Check sheet for the modelled part. Datum: model origin and axes. Units: mm. Face numbers are marked on the shaded views. A direction names the side the tool comes from. Round coordinates to 2 decimals unless told otherwise and drop trailing zeros. Loops run counter-clockwise (first coordinate to the right, second up) from the corner with the lowest first, then second, coordinate; pieces in that order, holes last. Notation, with made-up numbers: (83, 42) - (137, 42) arc R17 ccw to (137, 48) - close; hole circle Ø8 at (-35.5, 25). An arc over 180 degrees is marked (long way). Return JSON: item names as keys, results as strings.
Autodesk Inventor part; units mm, degrees
ref_plane "YZ Plane" through (0, 0, 0) normal (1, 0, 0) x (0, 1, 0)
ref_plane "XZ Plane" through (0, 0, 0) normal (0, 1, 0) x (-1, 0, 0)
ref_plane "XY Plane" through (0, 0, 0) normal (0, 0, 1) x (1, 0, 0)
sketch "Sketch1" plane through (0, 0, 0) normal (0, 0, 1) x (1, 0, 0)
  circle A0 centre (0, 0) radius 3
  dimension "d0" = 6
extrude "Extrusion1" add sketch "Sketch1" along normal blind 0.5
sketch "Sketch2" plane through (0, 0, 0.5) normal (0, 0, 1) x (1, 0, 0)
  circle A0 centre (0, 0) radius 3
  circle A1 centre (0, 0) radius 2
  dimension "d3" = 4
extrude "Extrusion2" add sketch "Sketch2" along normal blind 3 contours A1
hole "Hole1" at (0, 0, 3.5) direction (0, 0, -1) diameter 2 depth 3.5
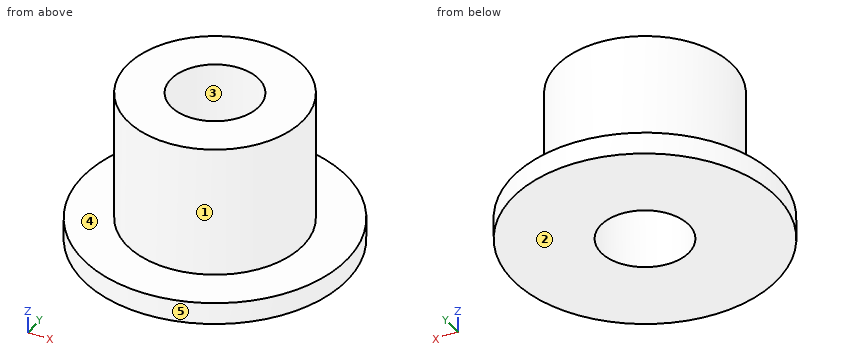
Q1. Tool access check on the marked faces 4 and 5. Record the directions out of +Z, -Z, +X, -X, +Y, -Y that give a thin tool (end or side, any length) a straight path to the whole face; none if there is none.
Answer key:
{"face 4": "+Z", "face 5": "+Z, -Z"}
Q2. Sectioned sample at B-B (y = 0.3). Enter the section's corners in (x, z), plus the area to 3 significant figures.
Answer key:
{"outline": "(-2.98, 0) - (-0.95, 0) - (-0.95, 3.5) - (-1.98, 3.5) - (-1.98, 0.5) - (-2.98, 0.5) - close; (0.95, 0) - (2.98, 0) - (2.98, 0.5) - (1.98, 0.5) - (1.98, 3.5) - (0.95, 3.5) - close", "area": "8.17 mm²"}
Q3. Sectioned sample at D-D (x = 1.9). Enter the section's corners in (y, z), plus the area to 3 significant figures.
Answer key:
{"outline": "(-2.32, 0) - (2.32, 0) - (2.32, 0.5) - (0.62, 0.5) - (0.62, 3.5) - (-0.62, 3.5) - (-0.62, 0.5) - (-2.32, 0.5) - close", "area": "6.07 mm²"}
Q4. Draft check along X on the marked faces 1, 2 and 3. Enter one of: released by +X, released by -X, zero draft, split by the parting line, or undercut.
Answer key:
{"face 1": "split by the parting line", "face 2": "zero draft", "face 3": "undercut"}
Q5. Scan lines: probe 1 along Y at (x, z) = (0, 2.7); probe 2 along Z at (x, y) = (-2, -2.2); probe 3 along X at (y, z) = (0.4, 2.5). Record each from-to range of solid material in increasing order. Write a range as [from, to].
Answer key:
{"probe 1": "y = [-2, -1], [1, 2]", "probe 2": "z = [0, 0.5]", "probe 3": "x = [-1.96, -0.92], [0.92, 1.96]"}
Q6. Sectioned sample at C-C (y = 1.35). Enter the section's corners in (x, z), plus the area to 3 significant figures.
Answer key:
{"outline": "(-2.68, 0) - (2.68, 0) - (2.68, 0.5) - (1.48, 0.5) - (1.48, 3.5) - (-1.48, 3.5) - (-1.48, 0.5) - (-2.68, 0.5) - close", "area": "11.5 mm²"}
Q7. Depth check by flat-ended pin: P1, Ø1, axis at y = -2, z = 1.5, coming from the -X side; P2, Ø1.5, axis at x = 2, z = 1.5, coming from the -Y side; P3, Ø1.5, axis at y = 1.5, z = 1.5, coming from the +X side; P4, Ø1.2, axis at x = 0, y = 0, coming from the -Z side. Enter the tip coordinate at first touch or a pass-through.
Answer key:
{"P1": "stops at x = -1.32", "P2": "stops at y = -1.56", "P3": "stops at x = 1.85", "P4": "passes through"}
Q8. Sectioned sample at A-A (x = 0). Enter the section's corners in (y, z).
Answer key:
{"outline": "(-3, 0) - (-1, 0) - (-1, 3.5) - (-2, 3.5) - (-2, 0.5) - (-3, 0.5) - close; (1, 0) - (3, 0) - (3, 0.5) - (2, 0.5) - (2, 3.5) - (1, 3.5) - close"}
